Design review of the part built by this model. Coordinates are the model's own, in mm. Coordinates: 2 decimals unless noted, no trailing zeros. Order: outer loops, then holes, each group sorted by start corner. A loop starts at its lowest first (then second) coordinate and runs counter-clockwise, first axis right, second up. Notation, with made-up numbers: M 67.25,13 L 83.25,13 A20 ccw 83.25,42 Z; hole C 34.5,9.25 d11. An arc over 180 degrees is marked long. Answer in a Markdown table with one row per item.
from build123d import *

# Parameters (mm, degrees)
SKETCH1_W           = 15
SKETCH1_H           = 20
BOSS_EXTRUDE1_DEPTH = 5


with BuildPart() as part:
    # Sketch1 → Boss-Extrude1 (new body)
    with BuildSketch(Plane.XY):
        Polygon((-54, -43), (-54, 37), (-52, 37), (-52, 39), (48, 39), (48, 37), (50, 37), (50, -43), (48, -43), (48, -45), (-52, -45), (-52, -43), align=None)
        with Locations((-7, 17)):
            Rectangle(SKETCH1_W, SKETCH1_H, mode=Mode.SUBTRACT)
        with Locations((-32, 17)):
            Rectangle(SKETCH1_W, SKETCH1_H, mode=Mode.SUBTRACT)
        with Locations((18, 17)):
            Rectangle(SKETCH1_W, SKETCH1_H, mode=Mode.SUBTRACT)
        with Locations((-7, -13)):
            Rectangle(SKETCH1_W, SKETCH1_H, mode=Mode.SUBTRACT)
        with Locations((18, -13)):
            Rectangle(SKETCH1_W, SKETCH1_H, mode=Mode.SUBTRACT)
        with Locations((-32, -13)):
            Rectangle(SKETCH1_W, SKETCH1_H, mode=Mode.SUBTRACT)
    extrude(amount=BOSS_EXTRUDE1_DEPTH)


solid = part.part
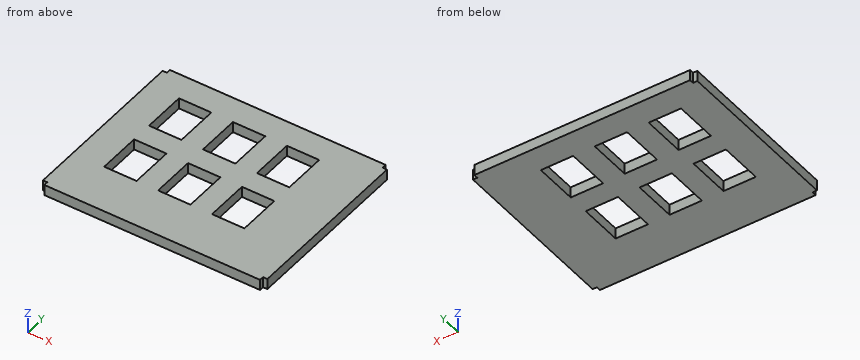
(1) Insertion check: pin 1 Ø1.6 at (y, z) = (38, 3.5) entering from +X. The pin has a flat end and moves straight along its axis. Give the tip position at first contact, or say it passes through.
Return value:
| item | result |
|---|---|
| pin 1 | stops at x = 48 |
(2) Add section B-B, the plane z = 0.8. Give the number of separate pieces and of enclosed holes in the cut face, and give its area (3 significant figures).
Return value:
| item | result |
|---|---|
| separate pieces | 1 |
| enclosed holes | 6 |
| area | 6,920 mm2 |
(3) For line 1 along Y through (x, z) = (-4.5, 3.4); line 2 along X through (y, z) = (-10, 2.7), list the stretches that pass through material, from the lowest coordinate up. Write a range as from..to.
Return value:
| item | result |
|---|---|
| line 1 | y = -45..-23, -3..7, 27..39 |
| line 2 | x = -54..-39.5, -24.5..-14.5, 0.5..10.5, 25.5..50 |
(4) Add section A-A, the plane y = 9.5. Give the boundary of the cut face in (x, z).
Return value:
| item | result |
|---|---|
| outline | M -54,0 L -39.5,0 L -39.5,5 L -54,5 Z; M -24.5,0 L -14.5,0 L -14.5,5 L -24.5,5 Z; M 0.5,0 L 10.5,0 L 10.5,5 L 0.5,5 Z; M 25.5,0 L 50,0 L 50,5 L 25.5,5 Z |
